from build123d import *

# Parameters (mm, degrees)
F0_W     = 50
F0_H     = 3
F1_DEPTH = 5
F3_DEPTH = 55.5734787771
F4_W     = 3
F4_H     = 0.2
F5_REACH = 58.5801380528


with BuildPart() as f1:
    # F0 (on Top) → F1 (new body)
    with BuildSketch(Plane.XY):
        Rectangle(F0_W, F0_H)
    extrude(amount=F1_DEPTH)


with BuildPart() as f1b:
    # F0 (on Top) → F1, piece 2 (new body)
    with BuildSketch(Plane.XY):
        Polygon((-26.5434872663, 24.0724787771), (-25, 21.5), (25, 51.5), (23.4565127337, 54.0724787771), align=None)
    extrude(amount=F1_DEPTH)


with BuildPart() as f3_tool:
    # F2 (on face) → F3 (new body, through all)
    with BuildSketch(Plane.XZ.offset(1.5)):
        Polygon((17.6366446762, 5), (-26.5434872663, 5), (-26.5434872663, 0.7142857143), (-19.1801319425, 0.7142857143), (-19.1801319425, 1.4285714286), (-11.8167766188, 1.4285714286), (-11.8167766188, 2.1428571429), (-4.453421295, 2.1428571429), (-4.453421295, 2.8571428571), (2.9099340287, 2.8571428571), (2.9099340287, 3.5714285714), (10.2732893525, 3.5714285714), (10.2732893525, 4.2857142857), (17.6366446762, 4.2857142857), align=None)
    extrude(amount=-F3_DEPTH)


with BuildPart() as f1_1:
    add(f1.part)

    # F3: cut by f3_tool
    add(f3_tool.part, mode=Mode.SUBTRACT)



with BuildPart() as f1b_1:
    add(f1b.part)

    # F3: cut by f3_tool
    add(f3_tool.part, mode=Mode.SUBTRACT)


with BuildPart() as f1_2:
    add(f1_1.part)

    add(f1b_1.part)  # F5 merges F1b
    f5_end = f1_2.faces().sort_by_distance((5.616262324, 43.3683285313, 1.7462125476))[0]
    # F4 (on face) → F5 (join, up to a face of the model that its end follows)
    with BuildSketch(Plane.XZ.offset(1.5)):
        with Locations((-22.0900659713, 0.6142857143)):
            Rectangle(F4_W, F4_H)
        with Locations((-15.4984542807, 1.3285714286)):
            Rectangle(F4_W, F4_H)
        with Locations((-8.1350989569, 2.0428571429)):
            Rectangle(F4_W, F4_H)
        with Locations((-0.7717436331, 2.7571428571)):
            Rectangle(F4_W, F4_H)
        with Locations((6.5916116906, 3.4714285714)):
            Rectangle(F4_W, F4_H)
        with Locations((13.9549670144, 4.1857142857)):
            Rectangle(F4_W, F4_H)
        with Locations((21.3183223381, 4.9)):
            Rectangle(F4_W, F4_H)
    f5_long = extrude(amount=-F5_REACH, mode=Mode.PRIVATE)
    add(split(f5_long, bisect_by=f5_end, keep=Keep.BOTTOM, mode=Mode.PRIVATE))


solid = f1_2.part
Here's how the part is built. I have some questions about the finished solid (model axes, mm). A direction names the side the tool comes from. Give positions to 0.01 mm unless a question says otherwise; leave off trailing zeros. Loops run counter-clockwise (first coordinate to the right, second up) from the corner with the lowest first, then second, coordinate; pieces in that order, holes last. Notation, with made-up numbers: (38.5, 69) -> (84.5, 69) arc R18 cw to (84.5, 104) -> close; hole circle Ø11 at (60, 47). An arc over 180 degrees is marked (long way). Answer as a JSON object with one key per item and string values. Group by question number.
Item 1: Will these pins go through, and if not, where does the flat tip stop? pin 1 (4 mm diameter, centred on x = -5.5, y = 34, fed in from +Z); pin 2 (1.5 mm diameter, centred on x = 14.5, y = 30.5, fed in from -Z); pin 3 (6 mm diameter, centred on x = 6.5, y = 23.5, fed in from +Z); pin 4 (10 mm diameter, centred on x = 15.5, y = 40.5, fed in from -Z).
Item 2: On a 3-axis mill with a long thin cutter (end or side, diameter ignored), from which of +Z, -Z, +X, -X, +Y, -Y can I reach the whole of each face in a straight line? I mean faces 1 (the flat face through (21, 33, 5)), 2 (the flat face through (-16, 15, 1.429)). Say none if no direction works.
Item 3: Imagine slicing it at A-A on y = 8. Write out the boundary of the cut face in (x, z).
Item 4: Imagine slicing it at B-B on x = -5.5. Write out the boundary of the cut face in (y, z).
Item 5: Thinking about a two-plate mould opening in Y: for faces 3 (the flat face through (-1, 19, 2.657)), 4 (the flat face through (0, 0, 0)), 5 (the flat face through (4.362, 42.616, 1.909)), 6 (the flat face through (5, -1.5, 2)), which applies, pulls with the +Y half, pulls with the -Y half, needs draft (parallel to the pull), parting line crosses it, or undercut?
Item 6: I need wall thicknesses on L1, parallel to Z at x = 14, y = 38.5; L2, parallel to Y at x = 15.5, z = 3.2; L3, parallel to Y at x = 20, z = 3.7. Which ranges of each line are inside material? Lowest first, please.
Item 7: Imagine slicing it at C-C on y = 34.5. Write out the boundary of the cut face in (x, z), then the cut area to 3 significant figures.
Answer list:
{
 "1": {"pin 1": "stops at z = 2.86", "pin 2": "stops at z = 4.09", "pin 3": "stops at z = 3.57", "pin 4": "stops at z = 0"},
 "2": {"face 1": "+Z, +X, -X, +Y, -Y", "face 2": "+Z, -X, +Y, -Y"},
 "3": {"outline": "(-23.59, 0.51) -> (-20.59, 0.51) -> (-20.59, 0.71) -> (-23.59, 0.71) -> close; (-17, 1.23) -> (-14, 1.23) -> (-14, 1.43) -> (-17, 1.43) -> close; (-9.64, 1.94) -> (-6.64, 1.94) -> (-6.64, 2.14) -> (-9.64, 2.14) -> close; (-2.27, 2.66) -> (0.73, 2.66) -> (0.73, 2.86) -> (-2.27, 2.86) -> close; (5.09, 3.37) -> (8.09, 3.37) -> (8.09, 3.57) -> (5.09, 3.57) -> close; (12.45, 4.09) -> (15.45, 4.09) -> (15.45, 4.29) -> (12.45, 4.29) -> close; (19.82, 4.8) -> (22.82, 4.8) -> (22.82, 5) -> (19.82, 5) -> close"},
 "4": {"outline": "(-1.5, 0) -> (1.5, 0) -> (1.5, 2.14) -> (-1.5, 2.14) -> close; (33.2, 0) -> (36.7, 0) -> (36.7, 2.14) -> (33.2, 2.14) -> close"},
 "5": {"face 3": "undercut", "face 4": "needs draft", "face 5": "pulls with the +Y half", "face 6": "pulls with the -Y half"},
 "6": {"L1": "z = 4.09 to 4.29", "L2": "y = -1.5 to 1.5, 45.8 to 49.3", "L3": "y = -1.5 to 1.5, 48.5 to 52"},
 "7": {"outline": "(-9.16, 0) -> (-3.33, 0) -> (-3.33, 2.86) -> (-4.45, 2.86) -> (-4.45, 2.14) -> (-9.16, 2.14) -> close; (-2.27, 2.66) -> (0.73, 2.66) -> (0.73, 2.86) -> (-2.27, 2.86) -> close; (5.09, 3.37) -> (8.09, 3.37) -> (8.09, 3.57) -> (5.09, 3.57) -> close; (12.45, 4.09) -> (15.45, 4.09) -> (15.45, 4.29) -> (12.45, 4.29) -> close; (19.82, 4.8) -> (22.82, 4.8) -> (22.82, 5) -> (19.82, 5) -> close", "area": "15.7 mm2"}
}
